from build123d import *

# Parameters (mm, degrees)
F0_R     = 7.5
F1_DEPTH = 30
F3_DEPTH = 7.5


with BuildPart() as f1:
    # F0 (on Right) → F1 (new body)
    with BuildSketch(Plane.YZ):
        Circle(F0_R)
    extrude(amount=F1_DEPTH)

    # F2 (on face) → F3 (join)
    with BuildSketch(Plane.YZ.offset(30)):
        with BuildLine():
            Line((17.09929, 10), (0, 10))
            ThreePointArc((0, 10), (-10, 0), (0, -10))
            Line((0, -10), (17.09929, -10))
            ThreePointArc((17.09929, -10), (27.09929, 0), (17.09929, 10))
        make_face()
    extrude(amount=F3_DEPTH)


solid = f1.part
Verification items for the finished model (mm, model axes). A direction names the side the tool comes from. Round coordinates to 2 decimals unless told otherwise and drop trailing zeros. Loops run counter-clockwise (first coordinate to the right, second up) from the corner with the lowest first, then second, coordinate; pieces in that order, holes last. Notation, with made-up numbers: (-3, -6.5) - (23, -6.5) arc R5 cw to (23, 2.5) - close; hole circle Ø10 at (46.5, 82). An arc over 180 degrees is marked (long way). Use one line per item in the form item = value.
1. Gauge pin test, flat ends, axial feed: pin 1 Ø12 at (x, z) = (27.5, -6) entering from -Y; pin 2 Ø4 at (x, y) = (11, 11) entering from +Z; pin 3 Ø1.5 at (x, y) = (24.5, 6) entering from +Z; pin 4 Ø12 at (x, z) = (5, 8) entering from +Y. Record the tip position at first contact, or that the pin passes through.
A:
pin_1 = -9.99
pin_2 = through
pin_3 = 5.36
pin_4 = 7.23
2. Section check A-A on z = 0. Record the cut outline in (x, y).
A:
outline = (0, -7.5) - (30, -7.5) - (30, -10) - (37.5, -10) - (37.5, 27.1) - (30, 27.1) - (30, 7.5) - (0, 7.5) - close
3. Section check B-B on y = 0.5. Record the cut outline in (x, z).
A:
outline = (0, -7.48) - (30, -7.48) - (30, -10) - (37.5, -10) - (37.5, 10) - (30, 10) - (30, 7.48) - (0, 7.48) - close
4. Section check D-D on y = 13.5. Record the cut outline in (x, z), and give its area (3 significant figures).
A:
outline = (30, -10) - (37.5, -10) - (37.5, 10) - (30, 10) - close
area = 150 mm²
5. Scan lines: probe 1 along X at (y, z) = (16.5, 7.75); probe 2 along Z at (x, y) = (18.5, 0); probe 3 along Y at (x, z) = (14.5, 5). Record each from-to range of solid material in increasing order.
A:
probe_1 = 30 to 37.5
probe_2 = -7.5 to 7.5
probe_3 = -5.59 to 5.59
6. Section check C-C on x = 23.5. Record the cut outline in (y, z).
A:
outline = circle Ø15 at (0, 0)
7. Access from +Z, -Z, +X, -X, +Y, -Y to the whole of each face (thin tool, end or side, straight path). Record for faces 1 (the cylindrical face through (14.79, -7.493, 0.33)), 2 (the flat face through (34, 8, -10)).
A:
face_1 = -X
face_2 = -Z, +X, -X, +Y, -Y
